Check sheet for the modelled part. Datum: model origin and axes. Units: mm. Face numbers are marked on the shaded views. A direction names the side the tool comes from. Round coordinates to 2 decimals unless told otherwise and drop trailing zeros. Write each loop counter-clockwise with the first axis right and the second up, starting at its lowest first coordinate (ties: lowest second). Pieces come first, ordered by that corner, then holes.
Item 1: Section check B-B, the plane x = 8. Record the cut outline in (y, z).
Item 2: Material ranges on line 1 along Z through (x, y) = (38, 21); line 2 along Z through (x, y) = (2, 38); line 3 along X through (y, z) = (20.5, -12.7) (3 decimals), recorded low to high.
Item 3: Release check for a two-part mould opening along Y. For the marked faces 5, 6 and 7 record: pulls with the +Y half, pulls with the -Y half, needs draft (parallel to the pull), parting line crosses it, or undercut.
Item 4: Section check D-D, the plane y = 23.5. Record the cut outline in (x, z) (3 decimals), plus the area to 3 significant figures.
Item 5: Section check A-A, the plane z = -28. Record the cut outline in (x, y), plus the area to 3 significant figures.
Item 6: Section check C-C, the plane x = 15. Record the cut outline in (y, z), plus the area to 3 significant figures.
Item 7: Depth check by flat-ended pin: pin 1 (5 mm diameter, centred on x = 15.5, z = -30, fed in from +Y); pin 2 (12 mm diameter, centred on y = 47, z = -22, fed in from +X); pin 3 (10 mm diameter, centred on x = 21.5, y = 31.5, fed in from +Z). Enter the tip coordinate at first touch or a pass-through.
Item 8: Set-up check for the marked faces 1, 2, 3 and 4: record each of +Z, -Z, +X, -X, +Y, -Y from which the full face is reachable in a straight line by a thin tool's end or side.
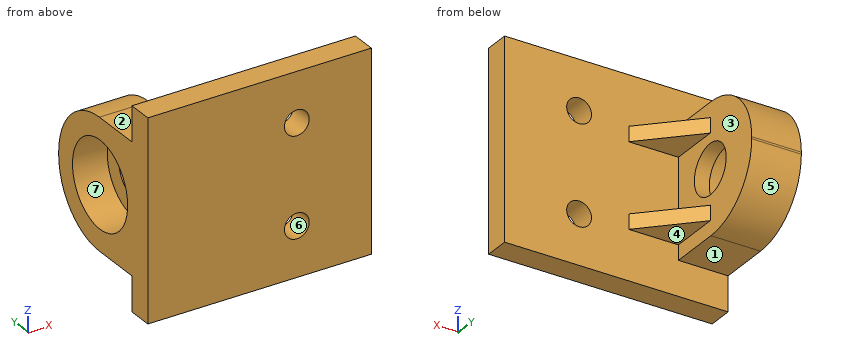
from build123d import *

# Parameters (mm, degrees)
SKETCH1_W           = 57.15
SKETCH1_H           = 50.8
BOSS_EXTRUDE1_DEPTH = 25.4
SKETCH2_W           = 50.8
SKETCH2_H           = 12.7
CUT_EXTRUDE1_DEPTH  = 81.572467382
SKETCH4_R           = 10.9982
BOSS_EXTRUDE2_DEPTH = 12.7
BOSS_EXTRUDE3_START = -3.81
SKETCH5_R           = 10.9982
SKETCH5_R_2         = 6.35
BOSS_EXTRUDE3_DEPTH = 3.81
SKETCH8_R           = 3.175
CUT_EXTRUDE2_DEPTH  = 94.962836271
SKETCH9_W           = 12.7
SKETCH9_H           = 3.81
BOSS_EXTRUDE5_DEPTH = 12.7
CUT_EXTRUDE3_DEPTH  = 88.749556124
CUT_EXTRUDE4_DEPTH  = 94.962836271


with BuildPart() as part:
    # Sketch1 → Boss-Extrude1 (new body)
    with BuildSketch(Plane(origin=(0, 0, 0), x_dir=(1, 0, 0), z_dir=(0, 1, 0))):
        with Locations((28.575, 25.4)):
            Rectangle(SKETCH1_W, SKETCH1_H)
    extrude(amount=BOSS_EXTRUDE1_DEPTH)

    # Sketch2 → Cut-Extrude1 (cut, through all)
    with BuildSketch(Plane.XY):
        with Locations((31.75, 12.7)):
            Rectangle(SKETCH2_W, SKETCH2_H)
    extrude(amount=-CUT_EXTRUDE1_DEPTH, mode=Mode.SUBTRACT)

    # Sketch4 → Boss-Extrude2 (add)
    with BuildSketch(Plane.ZY):
        with BuildLine():
            Line((-41.91, 25.4), (-8.89, 25.4))
            Line((-8.89, 25.4), (-8.89, 38.354))
            ThreePointArc((-8.89, 38.354), (-13.651272165, 49.848727835), (-25.146, 54.61))
            Line((-25.146, 54.61), (-25.654, 54.61))
            ThreePointArc((-25.654, 54.61), (-37.148727835, 49.848727835), (-41.91, 38.354))
            Line((-41.91, 38.354), (-41.91, 25.4))
        make_face()
        with Locations((-25.4, 38.1)):
            Circle(SKETCH4_R, mode=Mode.SUBTRACT)
    extrude(amount=-BOSS_EXTRUDE2_DEPTH)

    # Sketch5 → Boss-Extrude3 (add)
    with BuildSketch(Plane(origin=(12.7, 0, 0), x_dir=(0, 0, -1), z_dir=(1, 0, 0)).offset(BOSS_EXTRUDE3_START)):
        with Locations(Location((25.4, 38.1, 0), (0, 0, 180))):
            Circle(SKETCH5_R)
        with Locations((25.4, 38.1)):
            Circle(SKETCH5_R_2, mode=Mode.SUBTRACT)
    extrude(amount=BOSS_EXTRUDE3_DEPTH)

    # Sketch8 → Cut-Extrude2 (cut, through all)
    with BuildSketch(Plane.XZ):
        with Locations(Location((38.1, -38.1, 0), (0, 0, 270))):
            Circle(SKETCH8_R)
        with Locations(Location((38.1, -12.7, 0), (0, 0, 270))):
            Circle(SKETCH8_R)
    extrude(amount=-CUT_EXTRUDE2_DEPTH, mode=Mode.SUBTRACT)

    # Sketch9 → Boss-Extrude5 (add)
    with BuildSketch(Plane(origin=(0, 25.4, 0), x_dir=(1, 0, 0), z_dir=(0, 1, 0))):
        with Locations((19.05, 14.605)):
            Rectangle(SKETCH9_W, SKETCH9_H)
        with Locations((19.05, 36.195)):
            Rectangle(SKETCH9_W, SKETCH9_H)
    extrude(amount=BOSS_EXTRUDE5_DEPTH)

    # Sketch10 → Cut-Extrude3 (cut, through all)
    with BuildSketch(Plane.XY.offset(-12.7)):
        Polygon((25.4, 25.4), (25.4, 38.1), (12.7, 38.1), align=None)
    extrude(amount=-CUT_EXTRUDE3_DEPTH, mode=Mode.SUBTRACT)

    # Sketch11 → Cut-Extrude4 (cut, through all)
    with BuildSketch(Plane.XY):
        Polygon((6.35, 6.35), (6.35, 19.05), (0, 19.05), (0, 0), (57.15, 0), (57.15, 6.35), align=None)
    extrude(amount=-CUT_EXTRUDE4_DEPTH, mode=Mode.SUBTRACT)


solid = part.part
Values found:
1. outline: (19.05, -50.8) - (25.4, -50.8) - (25.4, -41.91) - (38.35, -41.91) arc R16.26 ccw to (54.61, -25.65) - (54.61, -25.15) arc R16.26 ccw to (38.35, -8.89) - (25.4, -8.89) - (25.4, 0) - (19.05, 0) - close; hole circle Ø22 at (38.1, -25.4)
2. line 1: z = -50.8 to -41.27, -34.93 to -15.87, -9.53 to 0
2. line 2: z = -41.91 to -36.4, -14.4 to -8.89
2. line 3: x = 0 to 34.925, 41.275 to 57.15
3. face 5: pulls with the +Y half
3. face 6: needs draft
3. face 7: undercut
4. outline: (0, -50.8) - (57.15, -50.8) - (57.15, 0) - (0, 0) - close; hole circle Ø6.35 at (38.1, -38.1); hole circle Ø6.35 at (38.1, -12.7)
4. area: 2,840 mm2
5. outline: (0, 19.05) - (57.15, 19.05) - (57.15, 25.4) - (12.7, 25.4) - (12.7, 32.31) - (8.89, 32.31) - (8.89, 27.41) - (0, 27.41) - close; (0, 48.79) - (8.89, 48.79) - (8.89, 43.89) - (12.7, 43.89) - (12.7, 54.44) - (0, 54.44) - close
5. area: 498 mm2
6. outline: (19.05, -50.8) - (25.4, -50.8) - (25.4, -38.1) - (35.8, -38.1) - (35.8, -34.29) - (25.4, -34.29) - (25.4, -16.51) - (35.8, -16.51) - (35.8, -12.7) - (25.4, -12.7) - (25.4, 0) - (19.05, 0) - close
6. area: 402 mm2
7. pin 1: stops at y = 25.4
7. pin 2: stops at x = 12.7
7. pin 3: stops at z = -12.7
8. face 1: -Z, +X, -X, +Y
8. face 2: +Z, +X, -X, +Y
8. face 3: +X, +Y
8. face 4: -Z, +X, +Y
